The listing builds one solid part. Answer for the finished solid, in the listing's coordinates (mm). Face numbers are marked on the shaded views. Coordinates: 2 decimals unless noted, no trailing zeros. Loops run counter-clockwise (first coordinate to the right, second up) from the corner with the lowest first, then second, coordinate; pieces in that order, holes last. Notation, with made-up numbers: (-5, 2) - (50, 2) arc R23 ccw to (50, 24) - close; hole circle Ø3 at (15.5, 55). An arc over 180 degrees is marked (long way). One line per question, with ' | ' between items.
from build123d import *

# Parameters (mm, degrees)
SKETCH1_W                 = 50.8
SKETCH1_H                 = 25.4
BOSS_EXTRUDE1_DEPTH       = 19.05
CUT_EXTRUDE1_DEPTH        = 19.05
F_6_CLEARANCE_HOLE1_D     = 3.7973
F_6_CLEARANCE_HOLE1_DEPTH = 11.43
F_6_32_TAPPED_HOLE1_D     = 2.7051


with BuildPart() as part:
    # Sketch1 → Boss-Extrude1 (new body)
    with BuildSketch(Plane.XY):
        with Locations((25.4, 12.7)):
            Rectangle(SKETCH1_W, SKETCH1_H)
    extrude(amount=BOSS_EXTRUDE1_DEPTH)

    # Sketch2 → Cut-Extrude1 (cut)
    with BuildSketch(Plane.XY.offset(19.05)):
        with BuildLine():
            Line((12.7, 13.97), (12.7, 11.43))
            Line((12.7, 11.43), (6.465334709, 11.43))
            ThreePointArc((6.465334709, 11.43), (13.338218788, 6.369389597), (19.0627, 12.7))
            ThreePointArc((19.0627, 12.7), (13.338218788, 19.030610403), (6.465334709, 13.97))
            Line((6.465334709, 13.97), (12.7, 13.97))
        make_face()
        with BuildLine():
            Line((6.465334709, 11.43), (12.7, 11.43))
            Line((12.7, 11.43), (12.7, 13.97))
            Line((12.7, 13.97), (6.465334709, 13.97))
            ThreePointArc((6.465334709, 13.97), (6.3373, 12.7), (6.465334709, 11.43))
        make_face()
        with BuildLine():
            Line((0, 11.43), (6.465334709, 11.43))
            ThreePointArc((6.465334709, 11.43), (6.3373, 12.7), (6.465334709, 13.97))
            Line((6.465334709, 13.97), (0, 13.97))
            Line((0, 13.97), (0, 11.43))
        make_face()
    extrude(amount=-CUT_EXTRUDE1_DEPTH, mode=Mode.SUBTRACT)

    # #6 Clearance Hole1
    with Locations(Plane(origin=(0, 25.4, 0), x_dir=(1, 0, 0), z_dir=(0, 1, 0))):
        with Locations((3.232667355, -9.525)):
            Hole(F_6_CLEARANCE_HOLE1_D / 2, depth=F_6_CLEARANCE_HOLE1_DEPTH)

    # #6-32 Tapped Hole1 (through all)
    with Locations(Plane(origin=(0, 11.43, 0), x_dir=(1, 0, 0), z_dir=(0, 1, 0))):
        with Locations((3.232667355, -9.525)):
            Hole(F_6_32_TAPPED_HOLE1_D / 2)


solid = part.part
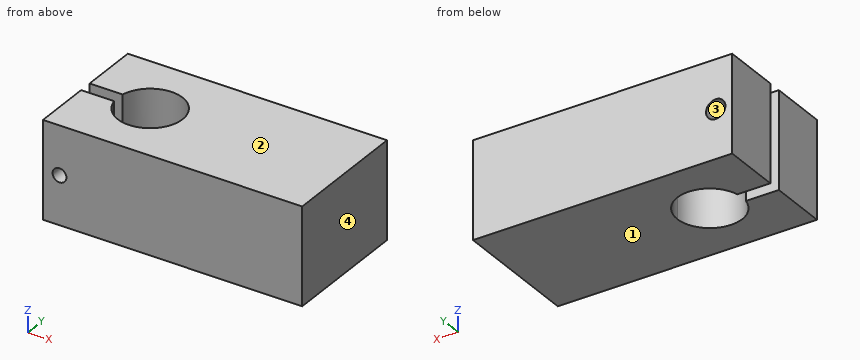
Item 1: The mould has two halves that part along Z. Classify the marked faces 1, 2, 3 and 4: pulls with the +Z half, pulls with the -Z half, needs draft (parallel to the pull), parting line crosses it, or undercut.
Taken from the geometry:
face 1: pulls with the -Z half | face 2: pulls with the +Z half | face 3: undercut | face 4: needs draft
Item 2: Find section C-C, the plane z = 4. Write down the section's boundary in (x, y).
Taken from the geometry:
outline: (0, 0) - (50.8, 0) - (50.8, 25.4) - (0, 25.4) - (0, 13.97) - (6.47, 13.97) arc R6.36 cw (long way) to (6.47, 11.43) - (0, 11.43) - close
Item 3: Find section A-A, the plane y = 18. State how many separate pieces and enclosed holes the cut face has, plus the area to 3 significant figures.
Taken from the geometry:
separate pieces: 2 | enclosed holes: 1 | area: 822 mm2
Item 4: Find the intervals of material crossed by line 1 (Y direction, x = 2, z = 15); line 2 (X direction, y = 17.25, z = 11.25); line 3 (Y direction, x = 10, z = 14.25), in increasing order. Write a range as [from, to].
Taken from the geometry:
line 1: y = [0, 11.43], [13.97, 25.4] | line 2: x = [0, 2.44], [4.03, 8.25], [17.15, 50.8] | line 3: y = [0, 6.94], [18.46, 25.4]
Item 5: Find section B-B, the plane z = 10.25. Write down the section's boundary in (x, y), plus the area to 3 significant figures.
Taken from the geometry:
outline: (0, 0) - (2.09, 0) - (2.09, 11.43) - (0, 11.43) - close; (0, 13.97) - (1.48, 13.97) - (1.48, 25.4) - (0, 25.4) - close; (4.37, 0) - (50.8, 0) - (50.8, 25.4) - (4.99, 25.4) - (4.99, 13.97) - (6.47, 13.97) arc R6.36 cw (long way) to (6.47, 11.43) - (4.37, 11.43) - close | area: 1,080 mm2
